```python
from build123d import *

# Parameters (mm, degrees)
SKETCH1_W           = 65
SKETCH1_H           = 100
SKETCH1_R           = 4
SKETCH1_R_2         = 1.6
BOSS_EXTRUDE1_DEPTH = 5
SKETCH3_R           = 3.5
CUT_EXTRUDE1_DEPTH  = 2


with BuildPart() as part:
    # Sketch1 → Boss-Extrude1 (new body)
    with BuildSketch(Plane(origin=(0, 0, 0), x_dir=(1, 0, 0), z_dir=(0, 1, 0))):
        Rectangle(SKETCH1_W, SKETCH1_H)
        with Locations((-25.4, -40)):
            Circle(SKETCH1_R, mode=Mode.SUBTRACT)
        with Locations((25.4, -40)):
            Circle(SKETCH1_R, mode=Mode.SUBTRACT)
        with Locations((25.4, -14.6)):
            Circle(SKETCH1_R, mode=Mode.SUBTRACT)
        with Locations((-25.4, -14.6)):
            Circle(SKETCH1_R, mode=Mode.SUBTRACT)
        with Locations((-17.5, 5.4)):
            Circle(SKETCH1_R_2, mode=Mode.SUBTRACT)
        with Locations((17.5, 37.4)):
            Circle(SKETCH1_R_2, mode=Mode.SUBTRACT)
        with Locations((-17.5, 37.4)):
            Circle(SKETCH1_R_2, mode=Mode.SUBTRACT)
        with Locations((17.5, 5.4)):
            Circle(SKETCH1_R_2, mode=Mode.SUBTRACT)
    extrude(amount=BOSS_EXTRUDE1_DEPTH)

    # Sketch3 → Cut-Extrude1 (cut)
    with BuildSketch(Plane.XZ):
        with Locations((-17.5, -5.4)):
            Circle(SKETCH3_R)
        with Locations((17.5, -5.4)):
            Circle(SKETCH3_R)
        with Locations((-17.5, -37.4)):
            Circle(SKETCH3_R)
        with Locations((17.5, -37.4)):
            Circle(SKETCH3_R)
    extrude(amount=-CUT_EXTRUDE1_DEPTH, mode=Mode.SUBTRACT)


solid = part.part
```
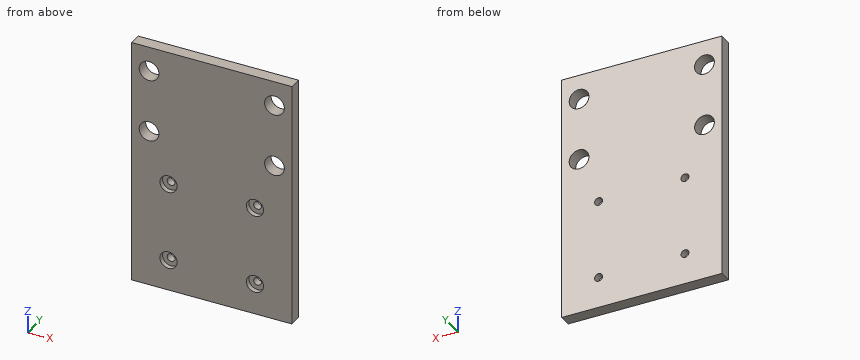
Check sheet for the modelled part. Datum: model origin and axes. Units: mm. Give positions to 0.01 mm unless a question says otherwise; leave off trailing zeros. Loops run counter-clockwise (first coordinate to the right, second up) from the corner with the lowest first, then second, coordinate; pieces in that order, holes last. Notation, with made-up numbers: (61.5, 40.25) - (90.5, 40.25) arc R32 ccw to (90.5, 71.25) - close; hole circle Ø2 at (-36, -24.75). An arc over 180 degrees is marked (long way). One line per question, with ' | ' between items. Start each with the question number.
1. Gauge pin test, flat end, axial feed: pin 1 Ø5.5 at (x, z) = (-17.5, -5.4) entering from -Y. Record the tip position at first contact, or that the pin passes through.
2. Cross-section at D-D, the plane x = -25.4. Enter the section's corners in (y, z), plus the area to 3 significant figures.
3. Material ranges on line 1 along X through (y, z) = (2.6, 14.6); line 2 along Z through (x, y) = (-18, 4.55); line 3 along X through (y, z) = (3.95, -37.4), recorded low to high. Write a range as [from, to].
4. Cross-section at A-A, the plane x = -17.5. Enter the section's corners in (y, z).
5. Cross-section at C-C, the plane y = 1.05. Give the number of separate pieces and of enclosed holes in the cut face, plus the area to 4 significant figures.
6. Cross-section at B-B, the plane z = 14.6. Enter the section's corners in (x, y).
Check result:
1) pin 1: stops at y = 2
2) outline: (0, -50) - (5, -50) - (5, 10.6) - (0, 10.6) - close; (0, 18.6) - (5, 18.6) - (5, 36) - (0, 36) - close; (0, 44) - (5, 44) - (5, 50) - (0, 50) - close | area: 420 mm2
3) line 1: x = [-32.5, -29.4], [-21.4, 21.4], [29.4, 32.5] | line 2: z = [-50, -38.92], [-35.88, -6.92], [-3.88, 50] | line 3: x = [-32.5, -19.1], [-15.9, 15.9], [19.1, 32.5]
4) outline: (0, -50) - (5, -50) - (5, -39) - (2, -39) - (2, -40.9) - (0, -40.9) - close; (0, -33.9) - (2, -33.9) - (2, -35.8) - (5, -35.8) - (5, -7) - (2, -7) - (2, -8.9) - (0, -8.9) - close; (0, -1.9) - (2, -1.9) - (2, -3.8) - (5, -3.8) - (5, 50) - (0, 50) - close
5) separate pieces: 1 | enclosed holes: 8 | area: 6,145 mm2
6) outline: (-32.5, 0) - (-29.4, 0) - (-29.4, 5) - (-32.5, 5) - close; (-21.4, 0) - (21.4, 0) - (21.4, 5) - (-21.4, 5) - close; (29.4, 0) - (32.5, 0) - (32.5, 5) - (29.4, 5) - close
